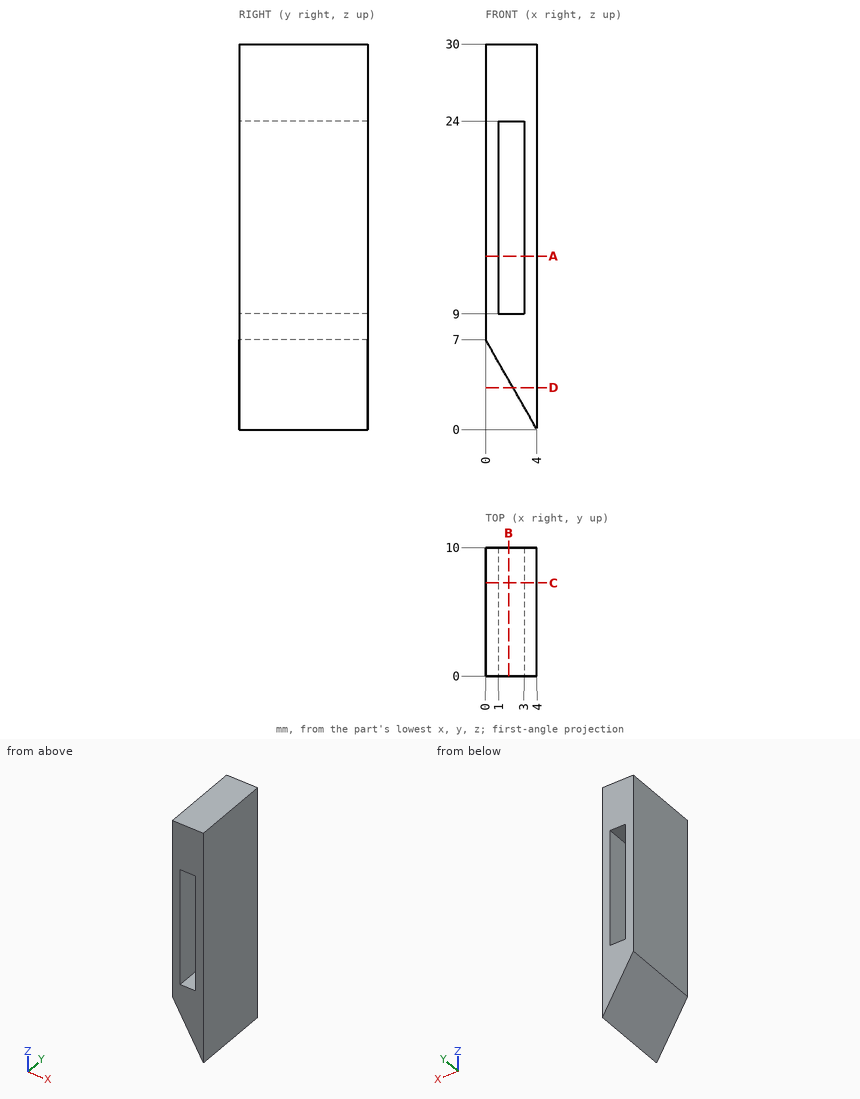
Input: dimensioned drawing with shaded views. Units: mm. Origin: part minimum x, y, z. Round coordinates to 2 decimals unless told otherwise and drop trailing zeros. Loops run counter-clockwise (first coordinate to the right, second up) from the corner with the lowest first, then second, coordinate; pieces in that order, holes last.
1) Pin query (flat end, axial travel): pin 1 (2 mm diameter, centred on x = 1.5, y = 7, fed in from -Z) (3 decimals); pin 2 (1 mm diameter, centred on x = 2, z = 22.5, fed in from +Y). Return the tip coordinate at first contact, or that it passes through.
Ans:
pin 1: stops at z = 2.625
pin 2: passes through
2) Section query B-B on x = 1.8. Return the cut outline in (y, z).
Ans:
outline: (0, 3.85) - (10, 3.85) - (10, 9) - (0, 9) - close; (0, 24) - (10, 24) - (10, 30) - (0, 30) - close
3) Section query C-C on y = 7.25. Return the cut outline in (x, z).
Ans:
outline: (0, 7) - (4, 0) - (4, 30) - (0, 30) - close; hole (1, 9) - (3, 9) - (3, 24) - (1, 24) - close
4) Section query A-A on z = 13.5. Return the cut outline in (x, y), plus the area to 3 significant figures.
Ans:
outline: (0, 0) - (1, 0) - (1, 10) - (0, 10) - close; (3, 0) - (4, 0) - (4, 10) - (3, 10) - close
area: 20.0 mm2
5) Section query D-D on z = 3.25. Return the cut outline in (x, y), plus the area to 3 significant figures.
Ans:
outline: (2.14, 0) - (4, 0) - (4, 10) - (2.14, 10) - close
area: 18.6 mm2
6) Material intervals for line 1 (X direction, y = 5.5, z = 16.75); line 2 (Z direction, x = 1.8, y = 9); line 3 (Z direction, x = 2, y = 4), sorted ascending.
Ans:
line 1: x = 0 to 1, 3 to 4
line 2: z = 3.85 to 9, 24 to 30
line 3: z = 3.5 to 9, 24 to 30
